Can you work these out from the model? Positions are in its coordinate system, mm. A direction names the side the tool comes from. Round coordinates to 2 decimals unless told otherwise and drop trailing zeros. Order: outer loops, then holes, each group sorted by start corner. A loop starts at its lowest first (then second) coordinate and runs counter-clockwise, first axis right, second up. Notation, with made-up numbers: (80.25, 48.25) - (126.25, 48.25) arc R20 cw to (126.25, 78.25) - close; hole circle Ø4 at (40, -22). An arc over 180 degrees is marked (long way). Write item = value, one per line.
from build123d import *

# Parameters (mm, degrees)
F2_R     = 5
F3_DEPTH = 15
F4_R     = 3
F5_DEPTH = 20
F6_R     = 2.9
F7_DEPTH = 20


with BuildPart() as f1:
    # F0 (on Front) → F1 (revolve)
    with BuildSketch(Plane.XZ):
        Polygon((7, 0), (0, 0), (0, -37), (5, -37), (5, -17), (7, -17), (10, -17), (10, -15), (7, -15), align=None)
    revolve(axis=Axis((0, 0, -18.5), (0, 0, 1)))

    # F2 (on face) → F3 (cut, through all)
    with BuildSketch(Plane.XY):
        Circle(F2_R)
    extrude(amount=-F3_DEPTH, mode=Mode.SUBTRACT)

    # F4 (on face) → F5 (cut, through all)
    with BuildSketch(Plane(origin=(0, 0, -37), x_dir=(1, 0, 0), z_dir=(0, 0, -1))):
        Circle(F4_R)
    extrude(amount=-F5_DEPTH, mode=Mode.SUBTRACT)


with BuildPart() as f7:
    # F6 (on face) → F7 (new body)
    with BuildSketch(Plane(origin=(0, 0, -37), x_dir=(1, 0, 0), z_dir=(0, 0, -1))):
        Circle(F6_R)
    extrude(amount=-F7_DEPTH)


solid = f1.part
(1) If we section it at D-D (z = -16.5): Write out the boundary of the cut face in (x, y), plus the area to 3 significant figures.
Computed:
outline = circle Ø20 at (0, 0)
area = 314 mm^2
(2) If we section it at A-A (y = 0): Write out the boundary of the cut face in (x, z).
Computed:
outline = (-10, -17) - (-5, -17) - (-5, -37) - (-3, -37) - (-3, -17) - (3, -17) - (3, -37) - (5, -37) - (5, -17) - (10, -17) - (10, -15) - (7, -15) - (7, 0) - (5, 0) - (5, -15) - (-5, -15) - (-5, 0) - (-7, 0) - (-7, -15) - (-10, -15) - close
(3) Will these pins go through, and if not, where does the flat tip stop? P1, Ø3, axis at x = -1, y = 1, coming from the +Z side; P2, Ø5, axis at x = 6.5, y = 5, coming from the -Z side; P3, Ø1.5, axis at y = 5, z = -5, coming from the +X side; P4, Ø6.5, axis at x = -0.5, y = -0.5, coming from the -Z side.
Computed:
P1 = -15
P2 = -17
P3 = 5.56
P4 = -37
(4) On a 3-axis mill with a long thin cutter (end or side, diameter ignored), from which of +Z, -Z, +X, -X, +Y, -Y can I reach the whole of each face in a straight line? I mean faces 1 (the face through (-2, 5, -17)), 2 (the face through (-1.08, -4.88, -7.4)), 3 (the face through (-2.17, -9.76, -15.99)). Say none if no direction works.
Computed:
face_1 = -Z
face_2 = +Z
face_3 = +Z, -Z
(5) If we section it at C-C (z = -5): Write out the boundary of the cut face in (x, y), plus the area to 3 significant figures.
Computed:
outline = circle Ø14 at (0, 0); hole circle Ø10 at (0, 0)
area = 75.4 mm^2
(6) If I drill on line 1 (Y direction, x = 0, z = -7); line 2 (Y direction, x = 0, z = -29.5); line 3 (Z direction, x = -2, y = -0.25), over which ranges is the centre line in solid material (lowest first)? Write a range as from..to.
Computed:
line_1 = -7..-5, 5..7
line_2 = -5..-3, 3..5
line_3 = -17..-15
(7) Thinking about a two-plate mould opening in Y: for faces 4 (the face through (0, 0, -17)), 5 (the face through (-1.08, -4.88, -26.86)), 6 (the face through (-2, 5, 0)), which applies, +Y half, -Y half, draft (parallel to the pull), parting line (faces both ways), or undercut?
Computed:
face_4 = undercut
face_5 = parting line
face_6 = draft
